Here's how the part is built. I have some questions about the finished solid (model axes, mm). A direction names the side the tool comes from. Coordinates: 2 decimals unless noted, no trailing zeros. Write each loop counter-clockwise with the first axis right and the second up, starting at its lowest first coordinate (ties: lowest second). Pieces come first, ordered by that corner, then holes. Notation, with made-up numbers: (2, -30.75) -> (60, -30.75) arc R26 ccw to (60, -14.75) -> close; hole circle Ø11 at (14.5, 60). An arc over 180 degrees is marked (long way). Use a Markdown table: item, result. Add a question column.
Item 1: If I drill on line 1 along Y through (x, z) = (-7.5, -11.45); line 2 along X through (y, z) = (-30.5, 10), over which ranges is the centre line in solid material (lowest first)? Write a range as from..to.
Item 2: Imagine slicing it at D-D, the plane z = 1. Write out the boundary of the cut face in (x, y).
Item 3: Imagine slicing it at A-A, the plane z = 7.5. Count the separate pieces of the cut face and the enclosed holes in it, and give its area (3 significant figures).
Item 4: Imagine slicing it at C-C, the plane y = 27.5. Write out the boundary of the cut face in (x, z).
Item 5: If we mould it in two halves opening along X, with no side actions, what happens to faces 3 (the cylindrical face through (11.76, -44.452, -7.066)), 4 (the flat face through (12.5, -1, 0)), 5 (the cylindrical face through (-7.066, 25.548, 11.74))? For each: pulls with the +X half, pulls with the -X half, needs draft (parallel to the pull), parting line crosses it, or undercut.
Item 6: On a 3-axis mill with a long thin cutter (end or side, diameter ignored), from which of +Z, -Z, +X, -X, +Y, -Y can I reach the whole of each face in a straight line? I mean faces 1 (the flat face through (-11, -1, 0)), 2 (the cylindrical face through (-7.066, 35.548, 11.74)). Say none if no direction works.
```python
from build123d import *

# Parameters (mm, degrees)
BOSS_EXTRUDE1_DEPTH      = 47.5
BOSS_EXTRUDE1_DEPTH_BACK = 47.5
SKETCH3_W                = 25
SKETCH3_H                = 25
SKETCH3_W_2              = 22
SKETCH3_H_2              = 22
SKETCH6_R                = 2
CUT_EXTRUDE3_DEPTH       = 25
SKETCH7_R                = 2
CUT_EXTRUDE4_DEPTH       = 25


with BuildPart() as part:
    # Sketch3 → Boss-Extrude1 (new, two sides: drawn at the far end of the back side and taken through both)
    with BuildSketch(Plane(origin=(0, 0, 0), x_dir=(1, 0, 0), z_dir=(0, 1, 0)).offset(-BOSS_EXTRUDE1_DEPTH_BACK)):
        Rectangle(SKETCH3_W, SKETCH3_H)
        Rectangle(SKETCH3_W_2, SKETCH3_H_2, mode=Mode.SUBTRACT)
    extrude(amount=BOSS_EXTRUDE1_DEPTH + BOSS_EXTRUDE1_DEPTH_BACK)

    # Sketch6 → Cut-Extrude3 (cut)
    with BuildSketch(Plane(origin=(12.5, 0, 0), x_dir=(0, 0, -1), z_dir=(1, 0, 0))):
        with Locations((7.5, -42.5)):
            Circle(SKETCH6_R)
        with Locations((7.5, -22.5)):
            Circle(SKETCH6_R)
        with Locations((-7.5, -42.5)):
            Circle(SKETCH6_R)
        with Locations((-7.5, -22.5)):
            Circle(SKETCH6_R)
        with Locations((7.5, -32.5)):
            Circle(SKETCH6_R)
        with Locations((-7.5, -32.5)):
            Circle(SKETCH6_R)
    extrude(amount=-CUT_EXTRUDE3_DEPTH, mode=Mode.SUBTRACT)

    # Sketch7 → Cut-Extrude4 (cut)
    with BuildSketch(Plane(origin=(0, 0, -12.5), x_dir=(-1, 0, 0), z_dir=(0, 0, -1))):
        with Locations((7.5, 37.5)):
            Circle(SKETCH7_R)
        with Locations((7.5, 27.5)):
            Circle(SKETCH7_R)
        with Locations((-7.5, 37.5)):
            Circle(SKETCH7_R)
        with Locations((-7.5, 27.5)):
            Circle(SKETCH7_R)
        with Locations((-7.5, 17.5)):
            Circle(SKETCH7_R)
        with Locations((7.5, 17.5)):
            Circle(SKETCH7_R)
    extrude(amount=-CUT_EXTRUDE4_DEPTH, mode=Mode.SUBTRACT)


solid = part.part
```
Ans:
| question | item | result |
|---|---|---|
| 1 | line 1 | y = -47.5..15.5, 19.5..25.5, 29.5..35.5, 39.5..47.5 |
| 1 | line 2 | x = -12.5..-11, 11..12.5 |
| 2 | outline | (-12.5, -47.5) -> (-11, -47.5) -> (-11, 47.5) -> (-12.5, 47.5) -> close; (11, -47.5) -> (12.5, -47.5) -> (12.5, 47.5) -> (11, 47.5) -> close |
| 3 | separate pieces | 8 |
| 3 | enclosed holes | 0 |
| 3 | area | 249 mm^2 |
| 4 | outline | (-12.5, -12.5) -> (-9.5, -12.5) -> (-9.5, -11) -> (-11, -11) -> (-11, 11) -> (-9.5, 11) -> (-9.5, 12.5) -> (-12.5, 12.5) -> close; (-5.5, -12.5) -> (5.5, -12.5) -> (5.5, -11) -> (-5.5, -11) -> close; (-5.5, 11) -> (5.5, 11) -> (5.5, 12.5) -> (-5.5, 12.5) -> close; (9.5, -12.5) -> (12.5, -12.5) -> (12.5, 12.5) -> (9.5, 12.5) -> (9.5, 11) -> (11, 11) -> (11, -11) -> (9.5, -11) -> close |
| 5 | face 3 | needs draft |
| 5 | face 4 | pulls with the +X half |
| 5 | face 5 | undercut |
| 6 | face 1 | +Y, -Y |
| 6 | face 2 | +Z, -Z |
